Check sheet for the modelled part. Datum: model origin and axes. Units: mm. A direction names the side the tool comes from. Give positions to 0.01 mm unless a question says otherwise; leave off trailing zeros. Order: outer loops, then holes, each group sorted by start corner. A loop starts at its lowest first (then second) coordinate and runs counter-clockwise, first axis right, second up.
Item 1: Sectioned sample at A-A on z = 3.1. Count the separate pieces of the cut face and the enclosed holes in it, and give its area (3 significant figures).
Item 2: Material ranges on line 1 along Y through (x, z) = (150, 2.6); line 2 along Y through (x, z) = (-20, 2.55); line 3 along X through (y, z) = (29, 1.9), recorded low to high.
Item 3: Gauge pin test, flat end, axial feed: P1, Ø3, axis at x = -99, z = 3, coming from the -Y side. Record the tip position at first contact, or that the pin passes through.
Item 4: Release check for a two-part mould opening along X. For faces 1 (the flat face through (-2, 21, 0)), 2 (the cylindrical face through (138, -1, 2)), 3 (the flat face through (-160, 20, 2)), 4 (the flat face through (160, 20, 2)) record: released by +X, released by -X, zero draft, split by the parting line, or undercut.
Item 5: Sectioned sample at B-B on x = 9. Record the boundary of the cut face in (y, z), and give its area (3 significant figures).
Item 6: Access from +Z, -Z, +X, -X, +Y, -Y to the whole of each face (thin tool, end or side, straight path). Record for faces 5 (the flat face through (2, 40, 2)), 6 (the cylindrical face through (-139, -2, 2)), 7 (the flat face through (-2, 21, 5)).
from build123d import *

# Parameters (mm, degrees)
BOSS_EXTRU_1_DEPTH = 5
D_GAGEMENT_M41_D   = 4.5
D_GAGEMENT_M42_D   = 4.5


with BuildPart() as part:
    # Esquisse1 → Boss.-Extru.1 (new body)
    with BuildSketch(Plane.XY):
        with BuildLine():
            Line((-135, 0), (135, 0))
            ThreePointArc((135, 0), (138.535533906, -1.464466094), (140, -5))
            Line((140, -5), (140, -10))
            ThreePointArc((140, -10), (150, -20), (160, -10))
            Line((160, -10), (160, 50))
            ThreePointArc((160, 50), (150, 60), (140, 50))
            Line((140, 50), (140, 45))
            ThreePointArc((140, 45), (138.535533906, 41.464466094), (135, 40))
            Line((135, 40), (-135, 40))
            ThreePointArc((-135, 40), (-138.535533906, 41.464466094), (-140, 45))
            Line((-140, 45), (-140, 50))
            ThreePointArc((-140, 50), (-150, 60), (-160, 50))
            Line((-160, 50), (-160, -10))
            ThreePointArc((-160, -10), (-150, -20), (-140, -10))
            Line((-140, -10), (-140, -5))
            ThreePointArc((-140, -5), (-138.535533906, -1.464466094), (-135, 0))
        make_face()
    extrude(amount=BOSS_EXTRU_1_DEPTH)

    # Dégagement M41 (through all)
    with Locations(Plane(origin=(0, 0, 0), x_dir=(-1, 0, 0), z_dir=(0, 0, -1))):
        with Locations((-150, -10), (150, 50), (150, -10), (-150, 50)):
            Hole(D_GAGEMENT_M41_D / 2)

    # Dégagement M42 (through all)
    with Locations(Plane(origin=(0, 0, 0), x_dir=(-1, 0, 0), z_dir=(0, 0, -1))):
        with Locations((20, 10), (-20, 10), (-20, 30), (20, 30)):
            Hole(D_GAGEMENT_M42_D / 2)


solid = part.part
Report:
1. separate pieces: 1
1. enclosed holes: 8
1. area: 14,100 mm2
2. line 1: y = -20 to -12.25, -7.75 to 47.75, 52.25 to 60
2. line 2: y = 0 to 7.75, 12.25 to 27.75, 32.25 to 40
2. line 3: x = -160 to -22.02, -17.98 to 17.98, 22.02 to 160
3. P1: stops at y = 0
4. face 1: zero draft
4. face 2: undercut
4. face 3: released by -X
4. face 4: released by +X
5. outline: (0, 0) - (40, 0) - (40, 5) - (0, 5) - close
5. area: 200 mm2
6. face 5: +Z, -Z, +Y
6. face 6: +Z, -Z, -Y
6. face 7: +Z, +X, -X, +Y, -Y
